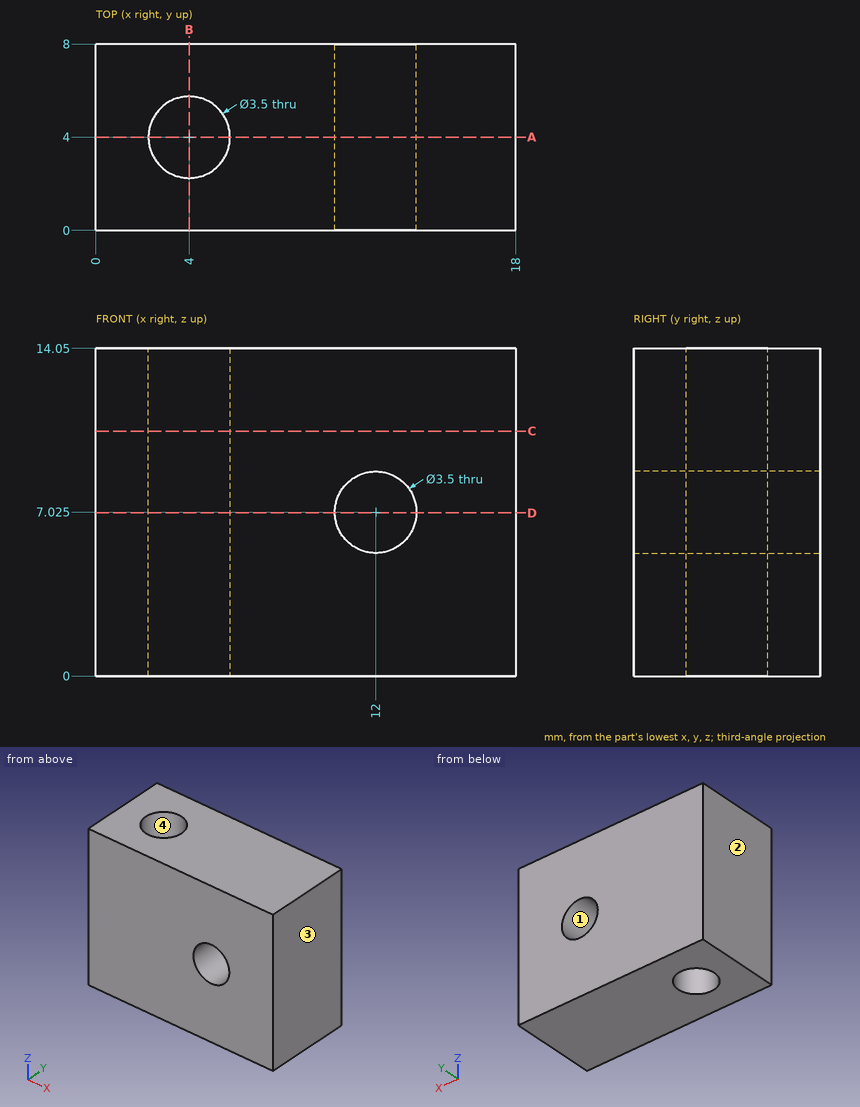
Here's the drawing with two shaded views (mm, measured from the low corner). I have some questions. Coordinates: 2 decimals unless noted, no trailing zeros. Write each loop counter-clockwise with the first axis right and the second up, starting at its lowest first coordinate (ties: lowest second). Pieces come first, ordered by that corner, then holes. Notation, with made-up numbers: (87, 40) -> (131, 40) arc R24 ccw to (131, 68) -> close; hole circle Ø7 at (-39, -18.75). An arc over 180 degrees is marked (long way). Use a Markdown table: item, result. Add a question column.
(1) We'd pull the mould along X, two halves only. Please class the marked faces 1, 2, 3 and 4: +X half, -X half, draft (parallel to the pull), parting line (faces both ways), or undercut.
(2) If we section it at C-C, the plane z = 10.5: Write out the boundary of the cut face in (x, y), and give its area (3 significant figures).
(3) Please list where these lines run through material, in increasing order: line 1 (Y direction, x = 4, z = 7); line 2 (X direction, y = 5, z = 7); line 3 (X direction, y = 2.5, z = 10.5).
(4) If we section it at A-A, the plane y = 4: Write out the boundary of the cut face in (x, z) (3 decimals).
(5) If we section it at B-B, the plane x = 4: Write out the boundary of the cut face in (y, z).
(6) I'm going to push a flat-ended pin straight in: P1, Ø3, axis at x = 4, y = 4, coming from the -Z side. Where does the tip first touch, or does it pass through?
(7) If we section it at D-D, the plane z = 7: Write out the boundary of the cut face in (x, y), and give its area (3 significant figures).
Outcome:
| question | item | result |
|---|---|---|
| 1 | face 1 | undercut |
| 1 | face 2 | -X half |
| 1 | face 3 | +X half |
| 1 | face 4 | undercut |
| 2 | outline | (0, 0) -> (18, 0) -> (18, 8) -> (0, 8) -> close; hole circle Ø3.5 at (4, 4) |
| 2 | area | 134 mm^2 |
| 3 | line 1 | y = 0 to 2.25, 5.75 to 8 |
| 3 | line 2 | x = 0 to 2.56, 5.44 to 10.25, 13.75 to 18 |
| 3 | line 3 | x = 0 to 3.1, 4.9 to 18 |
| 4 | outline | (0, 0) -> (2.25, 0) -> (2.25, 14.05) -> (0, 14.05) -> close; (5.75, 0) -> (18, 0) -> (18, 14.05) -> (5.75, 14.05) -> close; hole circle Ø3.5 at (12, 7.025) |
| 5 | outline | (0, 0) -> (2.25, 0) -> (2.25, 14.05) -> (0, 14.05) -> close; (5.75, 0) -> (8, 0) -> (8, 14.05) -> (5.75, 14.05) -> close |
| 6 | P1 | passes through |
| 7 | outline | (0, 0) -> (10.25, 0) -> (10.25, 8) -> (0, 8) -> close; (13.75, 0) -> (18, 0) -> (18, 8) -> (13.75, 8) -> close; hole circle Ø3.5 at (4, 4) |
| 7 | area | 106 mm^2 |
